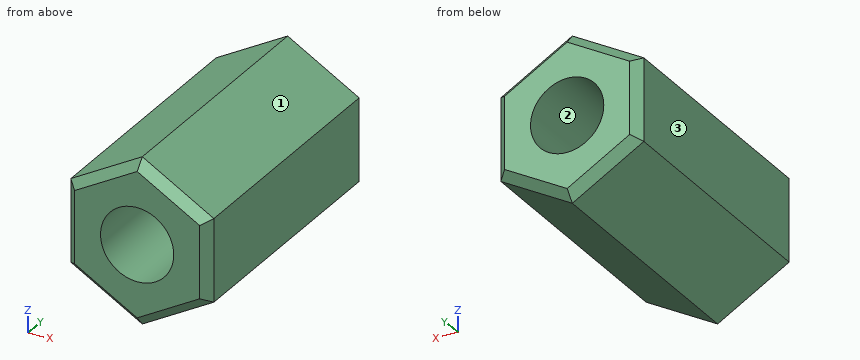
```python
from build123d import *

# Parameters (mm, degrees)
F1_DEPTH = 15
F2_D     = 4.1
F3_SIZE  = 0.5


with BuildPart() as f1:
    # F0 (on Front) → F1 (new body)
    with BuildSketch(Plane.XZ):
        Polygon((4, -2.3094010768), (4, 2.3094010768), (0, 4.6188021535), (-4, 2.3094010768), (-4, -2.3094010768), (0, -4.6188021535), align=None)
    extrude(amount=F1_DEPTH)

    # F2 (through all)
    with Locations(Plane(origin=(0, 0, 0), x_dir=(1, 0, 0), z_dir=(0, 1, 0))):
        with Locations((0, 0)):
            Hole(F2_D / 2)

    # F3
    f3_edges = [f1.edges().sort_by_distance(p)[0] for p in [
        (-2, 0, -3.464102),
        (-4, 0, 0),
        (-2, 0, 3.464102),
        (2, 0, 3.464102),
        (4, 0, 0),
        (2, 0, -3.464102),
        (4, -15, 0),
        (2, -15, 3.464102),
        (-2, -15, 3.464102),
        (-4, -15, 0),
        (-2, -15, -3.464102),
        (2, -15, -3.464102),
    ]]
    chamfer(f3_edges, length=F3_SIZE)


solid = f1.part
```
The listing builds one solid part. Answer for the finished solid, in the listing's coordinates (mm). Face numbers are marked on the shaded views. Give positions to 0.01 mm unless a question says otherwise; leave off trailing zeros. Order: outer loops, then holes, each group sorted by start corner. A loop starts at its lowest first (then second) coordinate and runs counter-clockwise, first axis right, second up. Notation, with made-up numbers: (-20, 30.5) -> (-7, 30.5) arc R12 cw to (-7, 35.5) -> close; hole circle Ø4 at (12.5, -3.5). An arc over 180 degrees is marked (long way). One line per item, written item: value.
1) A flat-ended cylindrical pin translates along its axis: P1, Ø2.5, axis at x = 0, z = 0, coming from the -Y side. Find the tip coordinate at first contact, or state that the pin passes through.
Reported:
P1: passes through
2) Find section A-A, the plane z = 0. Determine the outline of the cut face in (x, y).
Reported:
outline: (-4, -14.5) -> (-3.5, -15) -> (-2.05, -15) -> (-2.05, 0) -> (-3.5, 0) -> (-4, -0.5) -> close; (2.05, -15) -> (3.5, -15) -> (4, -14.5) -> (4, -0.5) -> (3.5, 0) -> (2.05, 0) -> close
3) Determine the mould class of the marked faces 1, 2 and 3 for opening direction Z: pulls with the +Z half, pulls with the -Z half, needs draft (parallel to the pull), parting line crosses it, or undercut.
Reported:
face 1: pulls with the +Z half
face 2: undercut
face 3: needs draft
4) Find section D-D, the plane z = 3.25. Determine the outline of the cut face in (x, y).
Reported:
outline: (-2.37, -14.5) -> (-1.37, -15) -> (1.37, -15) -> (2.37, -14.5) -> (2.37, -0.5) -> (1.37, 0) -> (-1.37, 0) -> (-2.37, -0.5) -> close
5) Find section C-C, the plane x = 0.75. Determine the outline of the cut face in (y, z).
Reported:
outline: (-15, -3.61) -> (-14.5, -4.19) -> (-0.5, -4.19) -> (0, -3.61) -> (0, -1.91) -> (-15, -1.91) -> close; (-15, 1.91) -> (0, 1.91) -> (0, 3.61) -> (-0.5, 4.19) -> (-14.5, 4.19) -> (-15, 3.61) -> close
6) Find the intervals of material crossed by line 1 (Z direction, x = 1, y = -6.5); line 2 (Z direction, x = -0.25, y = -2); line 3 (X direction, y = -13.25, z = -4), in increasing order.
Reported:
line 1: z = -4.04 to -1.79, 1.79 to 4.04
line 2: z = -4.47 to -2.03, 2.03 to 4.47
line 3: x = -1.07 to 1.07
7) Find section B-B, the plane y = -9.5. Determine the outline of the cut face in (x, z), plus the area to 3 significant figures.
Reported:
outline: (-4, -2.31) -> (0, -4.62) -> (4, -2.31) -> (4, 2.31) -> (0, 4.62) -> (-4, 2.31) -> close; hole circle Ø4.1 at (0, 0)
area: 42.2 mm^2
